Job drawing, mm, ordinate dimensions from the low corner. One solid piece. A direction names the side the tool comes from. Give positions to 0.01 mm unless a question says otherwise; leave off trailing zeros. Order: outer loops, then holes, each group sorted by start corner. A loop starts at its lowest first (then second) coordinate and runs counter-clockwise, first axis right, second up.
Item 1: Band-saw the part on B-B on x = 3. Give the cut face in (y, z), plus the area to 3 significant figures.
Item 2: Flat gauge pins, fed straight in: P1, Ø3, axis at x = 5, z = 3.5, coming from the +Y side; P2, Ø2, axis at y = 9.5, z = 2, coming from the +X side; P3, Ø1.5, axis at x = 7.5, z = 3.5, coming from the +Y side. Where does each tip first touch, or does it go through?
Item 3: Band-saw the part on C-C on y = 2.5. Give the cut face in (x, z), plus the area to 3 significant figures.
Item 4: Two-plate mould, pull along Y, no slides. Class the marked faces 3, 4, 5 and 6: released by +Y, released by -Y, zero draft, split by the parting line, or undercut.
Item 5: Wall check: L1, parallel to Z at x = 6.5, y = 5.75; L2, parallel to X at y = 2.25, z = 0.9; L3, parallel to X at y = 5, z = 4.8. Give the ranges that are in metal, low to high.
Item 6: Band-saw the part on A-A on y = 6.25. Give the cut face in (x, z).
Item 7: Band-saw the part on D-D on x = 9.5. Give the cut face in (y, z).
Item 8: Which spindle directions (+Z, -Z, +X, -X, +Y, -Y) get a long thin tool onto all of the face, cutting with end or side? Do the marked faces 1 and 2. Say none if no direction does.
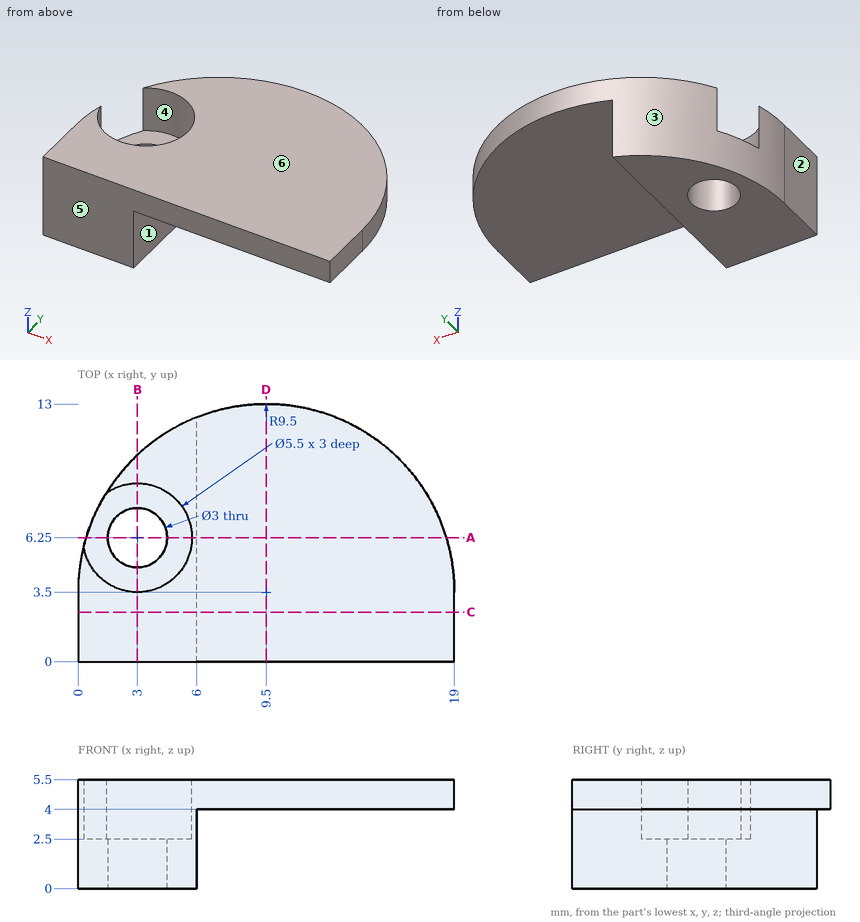
The answers:
1. outline: (0, 0) - (4.75, 0) - (4.75, 2.5) - (3.5, 2.5) - (3.5, 5.5) - (0, 5.5) - close; (7.75, 0) - (10.43, 0) - (10.43, 5.5) - (9, 5.5) - (9, 2.5) - (7.75, 2.5) - close
1. area: 33.4 mm2
2. P1: stops at y = 12.48
2. P2: stops at x = 6
2. P3: stops at y = 12.89
3. outline: (0, 0) - (6, 0) - (6, 4) - (19, 4) - (19, 5.5) - (0, 5.5) - close
3. area: 52.5 mm2
4. face 3: released by +Y
4. face 4: undercut
4. face 5: released by -Y
4. face 6: zero draft
5. L1: z = 4 to 5.5
5. L2: x = 0 to 6
5. L3: x = 0.12 to 0.55, 5.45 to 18.88
6. outline: (0.41, 0) - (1.5, 0) - (1.5, 2.5) - (0.41, 2.5) - close; (4.5, 0) - (6, 0) - (6, 4) - (18.59, 4) - (18.59, 5.5) - (5.75, 5.5) - (5.75, 2.5) - (4.5, 2.5) - close
7. outline: (0, 4) - (13, 4) - (13, 5.5) - (0, 5.5) - close
8. face 1: -Z, +X, +Y, -Y
8. face 2: +Z, -Z, -X, +Y, -Y
